```python
from build123d import *

# Parameters (mm, degrees)
SKETCH4_W           = 220
SKETCH4_H           = 220
BOSS_EXTRUDE2_DEPTH = 25.4
SKETCH5_R           = 3.2
CUT_EXTRUDE1_DEPTH  = 25.4
SKETCH7_R           = 3.2
CUT_EXTRUDE2_DEPTH  = 30
CUT_EXTRUDE4_START  = -30
SKETCH6_R           = 3.2
CUT_EXTRUDE4_DEPTH  = 30
SKETCH13_W          = 220
SKETCH13_H          = 25.4
BOSS_EXTRUDE3_DEPTH = 25


with BuildPart() as part:
    # Sketch4 → Boss-Extrude2 (new body)
    with BuildSketch(Plane(origin=(0, 0, 0), x_dir=(1, 0, 0), z_dir=(0, 1, 0))):
        with Locations((171.772904357, 21.481047821)):
            Rectangle(SKETCH4_W, SKETCH4_H)
    extrude(amount=BOSS_EXTRUDE2_DEPTH)

    # Sketch5 → Cut-Extrude1 (cut)
    with BuildSketch(Plane(origin=(0, 25.4, 0), x_dir=(1, 0, 0), z_dir=(0, 1, 0))):
        with Locations(Location((171.772904357, 21.481047821, 0), (0, 0, 270))):
            Circle(SKETCH5_R)
    extrude(amount=-CUT_EXTRUDE1_DEPTH, mode=Mode.SUBTRACT)

    # Sketch7 → Cut-Extrude2 (cut)
    with BuildSketch(Plane.ZY.offset(-61.772904357)):
        with Locations((-76.481047821, 12.7)):
            Circle(SKETCH7_R)
        with Locations((33.518952179, 12.7)):
            Circle(SKETCH7_R)
    extrude(amount=-CUT_EXTRUDE2_DEPTH, mode=Mode.SUBTRACT)

    # Sketch6 → Cut-Extrude4 (cut)
    with BuildSketch(Plane(origin=(281.772904357, 0, 0), x_dir=(0, 0, -1), z_dir=(1, 0, 0)).offset(CUT_EXTRUDE4_START)):
        with Locations(Location((-33.518952179, 12.7, 0), (0, 0, 180))):
            Circle(SKETCH6_R)
        with Locations(Location((76.481047821, 12.7, 0), (0, 0, 180))):
            Circle(SKETCH6_R)
    extrude(amount=CUT_EXTRUDE4_DEPTH, mode=Mode.SUBTRACT)

    # Sketch13 → Boss-Extrude3 (add)
    with BuildSketch(Plane.XY.offset(88.518952179)):
        with Locations((171.772904357, 12.7)):
            Rectangle(SKETCH13_W, SKETCH13_H)
    extrude(amount=BOSS_EXTRUDE3_DEPTH)


solid = part.part
```
Input: part model. Units: mm. Frame: model coordinates. A direction names the side the tool comes from. Coordinates: 2 decimals unless noted, no trailing zeros. Answer as a JSON object with one key per item and string values.
1. Access query for faces 4 (the face through (251.773, 13, -77)), 5 (the face through (91.773, 13, -77)), 6 (the face through (174.47, 12.88, -19.76)). Directions: +Z, -Z, +X, -X, +Y, -Y. A direction counts if a zero-diameter tool reaches every point of the face in a straight line with its end or side. Return the directions, or none.
Result set:
{"face 4": "+X", "face 5": "-X", "face 6": "+Y, -Y"}
2. First-contact query: P1, Ø7, axis at y = 13.5, z = -75.5, coming from the -X side; P2, Ø6, axis at y = 12.7, z = -76.48, coming from the -X side; P3, Ø5, axis at y = 12.7, z = 33.52, coming from the +X side. Flat tips, straight axial feed; report the tip coordinate or a pass-through.
Result set:
{"P1": "stops at x = 61.77", "P2": "stops at x = 91.77", "P3": "stops at x = 251.77"}
3. Material intervals for line 1 (Z direction, x = 268.5, y = 12.7); line 2 (X direction, y = 19.25, z = -21); line 3 (Z direction, x = 172, y = 14.75), sorted ascending. Write a range as from..to.
Result set:
{"line 1": "z = -131.48..-79.68, -73.28..30.32, 36.72..113.52", "line 2": "x = 61.77..168.61, 174.94..281.77", "line 3": "z = -131.48..-24.67, -18.29..113.52"}
4. Mould query, pull axis Z, two halves, no side actions, for faces 1 (the face through (251.773, 13, 33)), 2 (the face through (170, 13, 113.519)), 3 (the face through (61.773, 13, -11)). Classes: released by +Z, released by -Z, zero draft, split by the parting line, or undercut.
Result set:
{"face 1": "undercut", "face 2": "released by +Z", "face 3": "zero draft"}
